For this review, take the finished solid that the model builds, in its own axes (mm). Face numbers are marked on the shaded views. A direction names the side the tool comes from. Coordinates: 2 decimals unless noted, no trailing zeros. Write each loop counter-clockwise with the first axis right and the second up, starting at its lowest first coordinate (ties: lowest second). Pieces come first, ordered by that corner, then holes. Notation, with made-up numbers: (-34, 38) - (11, 38) arc R12 ccw to (11, 48) - close; hole circle Ø6 at (35.5, -35.75). An arc over 180 degrees is marked (long way). Use one line per item in the form item = value. Start each with the question number.
1) Mouldability with a two-part tool opening along X and no side actions: class the marked faces 1, 2, 3 and 4 as pulls with the +X half, pulls with the -X half, needs draft (parallel to the pull), parting line crosses it, or undercut.
2) For L1, parallel to X at y = 2.25, z = 3.5; L2, parallel to Z at x = 0, y = 7.9, list the stretches that pass through material, from the lowest coordinate up. Write a range as from..to.
3) We need section A-A (x = 0). Give the boundary of the cut face in (y, z) (3 decimals), plus the area to 3 significant figures.
4) We need section B-B (z = 0). Give the boundary of the cut face in (x, y) (3 decimals).
5) We need section C-C (y = 12.5). Count the separate pieces of the cut face and the enclosed holes in it, plus the area to 3 significant figures.
6) Insertion check: P1, Ø0.6, axis at x = 4, y = 13, coming from the +Z side; P2, Ø1.1, axis at y = 11.5, z = -4, coming from the -X side; P3, Ø2.5, axis at y = 10.5, z = 4, coming from the +X side. Each pin has a flat end and moves straight along its axis. Give the tip position at first contact, or say it passes through.
7) Tool access review of the marked faces 5, 6, 7, 8 and 9: name each direction out of +Z, -Z, +X, -X, +Y, -Y from which nothing blocks a thin tool from reaching the whole face with its end or side.
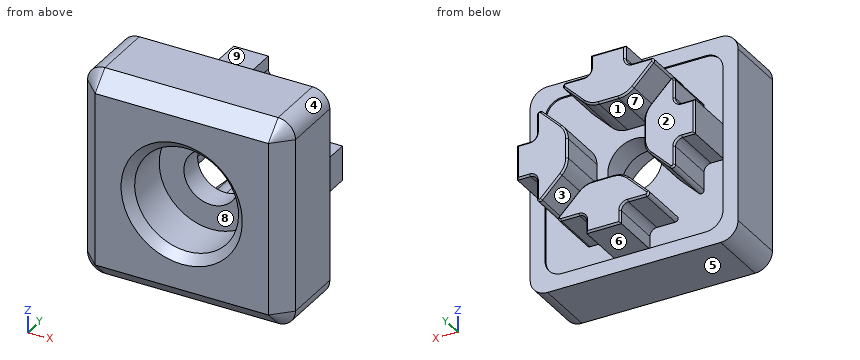
```python
from build123d import *

# Parameters (mm, degrees)
SKETCH1_W           = 24
SKETCH1_H           = 24
SKETCH1_R           = 3.15
BOSS_EXTRUDE1_DEPTH = 9
SKETCH2_W           = 20.55
SKETCH2_H           = 20.55
CUT_EXTRUDE1_DEPTH  = 0.2
SKETCH4_R           = 6
CUT_EXTRUDE2_DEPTH  = 6
FILLET1_R           = 2
CHAMFER1_SIZE       = 2
CHAMFER2_SIZE       = 1
BOSS_EXTRUDE2_DEPTH = 6
CHAMFER3_SIZE       = 0.2


with BuildPart() as part:
    # Sketch1 → Boss-Extrude1 (new body)
    with BuildSketch(Plane(origin=(0, 0, 0), x_dir=(1, 0, 0), z_dir=(0, 1, 0))):
        Rectangle(SKETCH1_W, SKETCH1_H)
        with Locations(Location((0, 0, 0), (0, 0, 270))):
            Circle(SKETCH1_R, mode=Mode.SUBTRACT)
    extrude(amount=BOSS_EXTRUDE1_DEPTH)

    # Sketch2 → Cut-Extrude1 (cut)
    with BuildSketch(Plane(origin=(0, 9, 0), x_dir=(1, 0, 0), z_dir=(0, 1, 0))):
        Rectangle(SKETCH2_W, SKETCH2_H)
    extrude(amount=-CUT_EXTRUDE1_DEPTH, mode=Mode.SUBTRACT)

    # Sketch4 → Cut-Extrude2 (cut)
    with BuildSketch(Plane.XZ):
        with Locations(Location((0, 0, 0), (0, 0, 270))):
            Circle(SKETCH4_R)
    extrude(amount=-CUT_EXTRUDE2_DEPTH, mode=Mode.SUBTRACT)

    # Fillet1
    fillet1_edges = [part.edges().sort_by_distance(p)[0] for p in [
        (-10.275, 8.9, 10.275),
        (-10.275, 8.9, -10.275),
        (10.275, 8.9, -10.275),
        (10.275, 8.9, 10.275),
        (-12, 4.5, -12),
        (12, 4.5, -12),
        (12, 4.5, 12),
        (-12, 4.5, 12),
    ]]
    fillet(fillet1_edges, radius=FILLET1_R)

    # Chamfer1
    chamfer1_edges = [part.edges().sort_by_distance(p)[0] for p in [
        (12, 0, 0),
        (-12, 0, 0),
        (0, 0, -12),
        (0, 0, 12),
        (11.414213562, 0, -11.414213562),
        (-11.414213562, 0, -11.414213562),
        (-11.414213562, 0, 11.414213562),
        (11.414213562, 0, 11.414213562),
    ]]
    chamfer(chamfer1_edges, length=CHAMFER1_SIZE - 0.0001)  # a hair under: the kernel refuses the full size

    # Chamfer2
    chamfer2_edges = [part.edges().sort_by_distance(p)[0] for p in [
        (0, 0, 6),
    ]]
    chamfer(chamfer2_edges, length=CHAMFER2_SIZE)

    # Sketch5 → Boss-Extrude2 (add)
    with BuildSketch(Plane(origin=(0, 8.8, 0), x_dir=(1, 0, 0), z_dir=(0, 1, 0))):
        with BuildLine():
            Line((7.9716, -5.195), (7.9716, -3.0868))
            ThreePointArc((7.9716, -3.0868), (8.207320463, -2.517720463), (8.7764, -2.282))
            Line((8.7764, -2.282), (10.275, -2.282))
            Line((10.275, -2.282), (10.275, 1.7218))
            Line((10.275, 1.7218), (8.7764, 1.7218))
            ThreePointArc((8.7764, 1.7218), (8.207320463, 1.957520463), (7.9716, 2.5266))
            Line((7.9716, 2.5266), (7.9716, 4.6348))
            ThreePointArc((7.9716, 4.6348), (7.762823537, 4.947256058), (7.394256487, 4.873943513))
            Line((7.394256487, 4.873943513), (5.139419138, 2.619106165))
            ThreePointArc((5.139419138, 2.619106165), (4.598094223, 1.808956178), (4.408006192, 0.853319111))
            Line((4.408006192, 0.853319111), (4.408006192, -1.413519111))
            ThreePointArc((4.408006192, -1.413519111), (4.598094223, -2.369156178), (5.139419138, -3.179306165))
            Line((5.139419138, -3.179306165), (7.394256487, -5.434143513))
            ThreePointArc((7.394256487, -5.434143513), (7.762823537, -5.507456058), (7.9716, -5.195))
        make_face()
        with BuildLine():
            Line((1.7218, -10.275), (-2.282, -10.275))
            Line((-2.282, -10.275), (-2.282, -8.7764))
            ThreePointArc((-2.282, -8.7764), (-2.517720463, -8.207320463), (-3.0868, -7.9716))
            Line((-3.0868, -7.9716), (-5.195, -7.9716))
            ThreePointArc((-5.195, -7.9716), (-5.507456058, -7.762823537), (-5.434143513, -7.394256487))
            Line((-5.434143513, -7.394256487), (-3.179306165, -5.139419138))
            ThreePointArc((-3.179306165, -5.139419138), (-2.369156178, -4.598094223), (-1.413519111, -4.408006192))
            Line((-1.413519111, -4.408006192), (0.853319111, -4.408006192))
            ThreePointArc((0.853319111, -4.408006192), (1.808956178, -4.598094223), (2.619106165, -5.139419138))
            Line((2.619106165, -5.139419138), (4.873943513, -7.394256487))
            ThreePointArc((4.873943513, -7.394256487), (4.947256058, -7.762823537), (4.6348, -7.9716))
            Line((4.6348, -7.9716), (2.5266, -7.9716))
            ThreePointArc((2.5266, -7.9716), (1.957520463, -8.207320463), (1.7218, -8.7764))
            Line((1.7218, -8.7764), (1.7218, -10.275))
        make_face()
        with BuildLine():
            Line((-10.275, -1.7218), (-10.275, 2.282))
            Line((-10.275, 2.282), (-8.7764, 2.282))
            ThreePointArc((-8.7764, 2.282), (-8.207320463, 2.517720463), (-7.9716, 3.0868))
            Line((-7.9716, 3.0868), (-7.9716, 5.195))
            ThreePointArc((-7.9716, 5.195), (-7.762823537, 5.507456058), (-7.394256487, 5.434143513))
            Line((-7.394256487, 5.434143513), (-5.139419138, 3.179306165))
            ThreePointArc((-5.139419138, 3.179306165), (-4.598094223, 2.369156178), (-4.408006192, 1.413519111))
            Line((-4.408006192, 1.413519111), (-4.408006192, -0.853319111))
            ThreePointArc((-4.408006192, -0.853319111), (-4.598094223, -1.808956178), (-5.139419138, -2.619106165))
            Line((-5.139419138, -2.619106165), (-7.394256487, -4.873943513))
            ThreePointArc((-7.394256487, -4.873943513), (-7.762823537, -4.947256058), (-7.9716, -4.6348))
            Line((-7.9716, -4.6348), (-7.9716, -2.5266))
            ThreePointArc((-7.9716, -2.5266), (-8.207320463, -1.957520463), (-8.7764, -1.7218))
            Line((-8.7764, -1.7218), (-10.275, -1.7218))
        make_face()
        with BuildLine():
            Line((-1.7218, 10.275), (2.282, 10.275))
            Line((2.282, 10.275), (2.282, 8.7764))
            ThreePointArc((2.282, 8.7764), (2.517720463, 8.207320463), (3.0868, 7.9716))
            Line((3.0868, 7.9716), (5.195, 7.9716))
            ThreePointArc((5.195, 7.9716), (5.507456058, 7.762823537), (5.434143513, 7.394256487))
            Line((5.434143513, 7.394256487), (3.179306165, 5.139419138))
            ThreePointArc((3.179306165, 5.139419138), (2.369156178, 4.598094223), (1.413519111, 4.408006192))
            Line((1.413519111, 4.408006192), (-0.853319111, 4.408006192))
            ThreePointArc((-0.853319111, 4.408006192), (-1.808956178, 4.598094223), (-2.619106165, 5.139419138))
            Line((-2.619106165, 5.139419138), (-4.873943513, 7.394256487))
            ThreePointArc((-4.873943513, 7.394256487), (-4.947256058, 7.762823537), (-4.6348, 7.9716))
            Line((-4.6348, 7.9716), (-2.5266, 7.9716))
            ThreePointArc((-2.5266, 7.9716), (-1.957520463, 8.207320463), (-1.7218, 8.7764))
            Line((-1.7218, 8.7764), (-1.7218, 10.275))
        make_face()
    extrude(amount=BOSS_EXTRUDE2_DEPTH)

    # Chamfer3
    chamfer3_edges = [part.edges().sort_by_distance(p)[0] for p in [
        (-1.957520463, 14.8, -8.207320463),
        (2.517720463, 14.8, -8.207320463),
        (-1.7218, 14.8, -9.5257),
        (-3.5807, 14.8, -7.9716),
        (-4.947256058, 14.8, -7.762823537),
        (-3.746524839, 14.8, -6.266837812),
        (-1.808956178, 14.8, -4.598094223),
        (0.2801, 14.8, -4.408006192),
        (2.369156178, 14.8, -4.598094223),
        (4.306724839, 14.8, -6.266837812),
        (5.507456058, 14.8, -7.762823537),
        (4.1409, 14.8, -7.9716),
        (2.282, 14.8, -9.5257),
        (0.2801, 14.8, -10.275),
        (-8.207320463, 14.8, 1.957520463),
        (-8.207320463, 14.8, -2.517720463),
        (-9.5257, 14.8, 1.7218),
        (-7.9716, 14.8, 3.5807),
        (-7.762823537, 14.8, 4.947256058),
        (-6.266837812, 14.8, 3.746524839),
        (-4.598094223, 14.8, 1.808956178),
        (-4.408006192, 14.8, -0.2801),
        (-4.598094223, 14.8, -2.369156178),
        (-6.266837812, 14.8, -4.306724839),
        (-7.762823537, 14.8, -5.507456058),
        (-7.9716, 14.8, -4.1409),
        (-9.5257, 14.8, -2.282),
        (-10.275, 14.8, -0.2801),
        (1.957520463, 14.8, 8.207320463),
        (-2.517720463, 14.8, 8.207320463),
        (1.7218, 14.8, 9.5257),
        (3.5807, 14.8, 7.9716),
        (4.947256058, 14.8, 7.762823537),
        (3.746524839, 14.8, 6.266837812),
        (1.808956178, 14.8, 4.598094223),
        (-0.2801, 14.8, 4.408006192),
        (-2.369156178, 14.8, 4.598094223),
        (-4.306724839, 14.8, 6.266837812),
        (-5.507456058, 14.8, 7.762823537),
        (-4.1409, 14.8, 7.9716),
        (-2.282, 14.8, 9.5257),
        (-0.2801, 14.8, 10.275),
        (8.207320463, 14.8, -1.957520463),
        (8.207320463, 14.8, 2.517720463),
        (9.5257, 14.8, -1.7218),
        (7.9716, 14.8, -3.5807),
        (7.762823537, 14.8, -4.947256058),
        (6.266837812, 14.8, -3.746524839),
        (4.598094223, 14.8, -1.808956178),
        (4.408006192, 14.8, 0.2801),
        (4.598094223, 14.8, 2.369156178),
        (6.266837812, 14.8, 4.306724839),
        (7.762823537, 14.8, 5.507456058),
        (7.9716, 14.8, 4.1409),
        (9.5257, 14.8, 2.282),
        (10.275, 14.8, 0.2801),
    ]]
    chamfer(chamfer3_edges, length=CHAMFER3_SIZE)


solid = part.part
```
Determined:
q1.face_1 = undercut
q1.face_2 = needs draft
q1.face_3 = undercut
q1.face_4 = pulls with the +X half
q2.L1 = -12..-4.87, 4.87..12
q2.L2 = -12..-3.15, 3.15..12
q3.outline = (0, -10) - (2, -12) - (9, -12) - (9, -10.275) - (14.6, -10.275) - (14.8, -10.075) - (14.8, -4.608) - (14.6, -4.408) - (8.8, -4.408) - (8.8, -3.15) - (6, -3.15) - (6, -6) - (1, -6) - (0, -7) - close; (0, 7) - (1, 6) - (6, 6) - (6, 3.15) - (8.8, 3.15) - (8.8, 4.408) - (14.6, 4.408) - (14.8, 4.608) - (14.8, 10.075) - (14.6, 10.275) - (9, 10.275) - (9, 12) - (2, 12) - (0, 10) - close
q3.area = 188 mm²
q4.outline = (-12, 2) - (-10, 0) - (-7, 0) - (-6, 1) - (-6, 6) - (-3.15, 6) - (-3.15, 8.8) - (-4.408, 8.8) - (-4.408, 14.6) - (-4.608, 14.8) - (-10.075, 14.8) - (-10.275, 14.6) - (-10.275, 9) - (-12, 9) - close; (3.15, 6) - (6, 6) - (6, 1) - (7, 0) - (10, 0) - (12, 2) - (12, 9) - (10.275, 9) - (10.275, 14.6) - (10.075, 14.8) - (4.608, 14.8) - (4.408, 14.6) - (4.408, 8.8) - (3.15, 8.8) - close
q5.separate_pieces = 4
q5.enclosed_holes = 0
q5.area = 148 mm²
q6.P1 = 7.97
q6.P2 = -7.97
q6.P3 = 8.05
q7.face_5 = -Z, +X, -X, +Y, -Y
q7.face_6 = -Z, +X, -X, +Y
q7.face_7 = +Y
q7.face_8 = -Y
q7.face_9 = +Z, +X, -X, +Y
